Check sheet for the modelled part. Datum: model origin and axes. Units: mm. Face numbers are marked on the shaded views. A direction names the side the tool comes from. Coordinates: 2 decimals unless noted, no trailing zeros. Order: outer loops, then holes, each group sorted by start corner. A loop starts at its lowest first (then second) coordinate and runs counter-clockwise, first axis right, second up.
from build123d import *

# Parameters (mm, degrees)
F1_DEPTH = 10


# Not quite as in the source:
# - a feature of the source that left no trace in its solid (it failed there, or was rolled back) is left out


with BuildPart() as f1:
    # F0 (on Front) → F1 (new body)
    with BuildSketch(Plane.XZ):
        Polygon((-54.1052184999, 47.8023849428), (-57.6798580587, 47.8023849428), (-57.6798580587, -27.2650625557), (-60.5125948787, -31.5141640604), (-60.5125948787, -46.9525642693), (-54.1052184999, -47.0233857632), (-54.1052184999, -31.1857834458), (-39.3331050873, -31.1857834458), (-39.3331050873, -46.9423271716), (-29.3199270964, -46.9423271716), (-29.3199270964, -21.3033463806), (-39.9415493011, -7.9316543415), (-39.9415493011, 17.7926272154), (-29.6685695648, 28.9044026285), (-29.6685695648, 47.8023849428), (-32.8597128391, 47.8023849428), (-32.8597128391, 28.9044026285), (-39.9415493011, 21.5739104897), (-39.9415493011, 47.8023849428), (-43.3408282697, 47.8023849428), (-43.3408282697, 24.3615116924), (-54.1052184999, 24.3615116924), align=None)
        Polygon((-54.1052184999, -7.0560085587), (-43.3408282697, -7.0560085587), (-39.3331050873, -12.5158438459), (-39.3331050873, -27.2650625557), (-54.1052184999, -27.2650625557), align=None, mode=Mode.SUBTRACT)
        Polygon((-43.3408282697, 6.7588053644), (-43.3408282697, -1.2844107114), (-43.3408282697, -4.0514403954), (-54.1052184999, -4.0514403954), (-54.1052184999, 6.7588053644), align=None, mode=Mode.SUBTRACT)
        Polygon((-43.3408282697, 21.1618710309), (-43.3408282697, 11.6142081097), (-43.3408282697, 10.3236073628), (-54.1052184999, 10.3236073628), (-54.1052184999, 21.1618710309), align=None, mode=Mode.SUBTRACT)
    extrude(amount=F1_DEPTH)


solid = f1.part
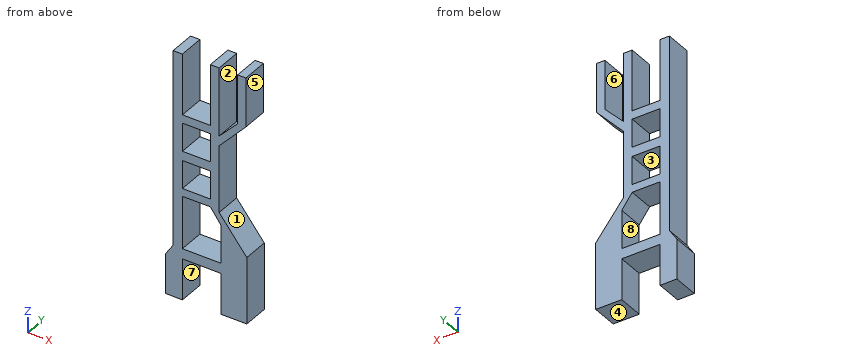
(1) Tool access check on the marked faces 5, 6, 7 and 8. Record the directions out of +Z, -Z, +X, -X, +Y, -Y that give a thin tool (end or side, any length) a straight path to the whole face; none if there is none.
Filled in:
face 5: +Z, +X, +Y, -Y
face 6: +Z, +Y, -Y
face 7: -Z, +Y, -Y
face 8: +Y, -Y
(2) Release check for a two-part mould opening along Z. For the marked faces 1, 2, 3 and 4 record: +Z half, -Z half, draft (parallel to the pull), parting line (faces both ways), or undercut.
Filled in:
face 1: undercut
face 2: draft
face 3: undercut
face 4: -Z half
(3) Thickness scan on probe 1 along Z at (x, y) = (-44, -2.75); probe 2 along X at (y, z) = (-5.25, 42.5); probe 3 along X at (y, z) = (-0.25, -35.5). Record the ranges inside material, lowest first.
Filled in:
probe 1: z = -31.19 to -27.27, -7.06 to -4.05, 6.76 to 10.32, 21.16 to 24.36
probe 2: x = -57.68 to -54.11, -43.34 to -39.94, -32.86 to -29.67
probe 3: x = -60.51 to -54.11, -39.33 to -29.32
(4) Cross-section at B-B (x = -32). Enter the section's corners in (y, z).
Filled in:
outline: (-10, -46.94) - (0, -46.94) - (0, -17.93) - (-10, -17.93) - close; (-10, 26.38) - (0, 26.38) - (0, 47.8) - (-10, 47.8) - close
(5) Cross-section at A-A (z = -34). Enter the section's corners in (x, y), and give its area (3 significant figures).
Filled in:
outline: (-60.51, -10) - (-54.11, -10) - (-54.11, 0) - (-60.51, 0) - close; (-39.33, -10) - (-29.32, -10) - (-29.32, 0) - (-39.33, 0) - close
area: 164 mm2
(6) Cross-section at C-C (y = -2.5). Count the separate pieces of the cut face and the enclosed holes in it, and give its area (3 significant figures).
Filled in:
separate pieces: 1
enclosed holes: 3
area: 1,160 mm2
(7) Go/stop test with flat-tipped pins: P1, Ø3, axis at y = -6, z = -1, coming from the +X side; P2, Ø6, axis at x = -47, y = -9, coming from the -Z side; P3, Ø5, axis at y = -5, z = 34, coming from the +X side; P4, Ø2, axis at x = -45.5, z = 12, coming from the +Y side. Record where each tip stops, or that it passes through.
Filled in:
P1: stops at x = -39.94
P2: stops at z = -31.19
P3: stops at x = -29.67
P4: passes through
